Design review of the part built by this model. Coordinates are the model's own, in mm. A direction names the side the tool comes from. Coordinates: 2 decimals unless noted, no trailing zeros. Loops run counter-clockwise (first coordinate to the right, second up) from the corner with the lowest first, then second, coordinate; pieces in that order, holes last. Notation, with made-up numbers: M -24.5,31 L -1.5,31 A17 cw -1.5,60 Z; hole C 0,44.5 d4. An arc over 180 degrees is marked long. One line per item, written item: value.
```python
from build123d import *

# Parameters (mm, degrees)
BOSS_EXTRUDE1_DEPTH      = 14
BOSS_EXTRUDE1_DEPTH_BACK = 14
BOSS_EXTRUDE3_DEPTH      = 14.084146884
CUT_EXTRUDE1_START       = 11.1
CUT_EXTRUDE1_DEPTH       = 22.2
SKETCH7_R                = 8.05
CUT_EXTRUDE2_DEPTH       = 3
SKETCH8_R                = 3
CUT_EXTRUDE4_DEPTH       = 50.90760018
FILLET4_R                = 2
CHAMFER6_SIZE            = 1


with BuildPart() as part:
    # Sketch1 → Boss-Extrude1 (new, two sides: drawn at the far end of the back side and taken through both)
    with BuildSketch(Plane(origin=(0, 0, 0), x_dir=(0, 0, -1), z_dir=(1, 0, 0)).offset(-BOSS_EXTRUDE1_DEPTH_BACK)):
        Polygon((0, 0), (14.084146884, 0), (14.084146884, 26.488427786), align=None)
    extrude(amount=BOSS_EXTRUDE1_DEPTH + BOSS_EXTRUDE1_DEPTH_BACK)

    # Sketch5 → Boss-Extrude3 (add)
    with BuildSketch(Plane.XY):
        Polygon((14, -10), (14, 0), (11.1, 0), (11.1, -14), (31, -14), (31, -10), align=None)
        Polygon((-14, 0), (-14, -10), (-31, -10), (-31, -14), (-11.1, -14), (-11.1, 0), align=None)
    extrude(amount=-BOSS_EXTRUDE3_DEPTH)

    # Sketch6 → Cut-Extrude1 (cut)
    with BuildSketch(Plane(origin=(0, 0, 0), x_dir=(0, 0, -1), z_dir=(1, 0, 0)).offset(CUT_EXTRUDE1_START)):
        Polygon((14.084146884, 0), (2.126837727, 0), (14.084146884, 22.488427786), align=None)
    extrude(amount=-CUT_EXTRUDE1_DEPTH, mode=Mode.SUBTRACT)

    # Sketch7 → Cut-Extrude2 (cut)
    with BuildSketch(Plane(origin=(0, 0, 0), x_dir=(1, 0, 0), z_dir=(0, 0.4694715627858856, 0.8829475928589298))):
        with Locations(Location((0, 15, 0), (0, 0, 270))):
            Circle(SKETCH7_R)
    extrude(amount=-CUT_EXTRUDE2_DEPTH, mode=Mode.SUBTRACT)

    # Sketch8 → Cut-Extrude4 (cut, through all)
    with BuildSketch(Plane(origin=(0, -10, 0), x_dir=(1, 0, 0), z_dir=(0, 1, 0))):
        with Locations(Location((22, 7.042073442, 0), (0, 0, 270))):
            Circle(SKETCH8_R)
        with Locations(Location((-22, 7.042073442, 0), (0, 0, 90))):
            Circle(SKETCH8_R)
    extrude(amount=-CUT_EXTRUDE4_DEPTH, mode=Mode.SUBTRACT)

    # Fillet4
    fillet4_edges = [part.edges().sort_by_distance(p)[0] for p in [
        (14, -10, -7.042073442),
        (-14, -10, -7.042073442),
        (-11.1, 0, -1.063418863),
        (11.1, 0, -1.063418863),
        (11.1, 11.244213893, -8.105492305),
        (-11.1, 11.244213893, -8.105492305),
    ]]
    fillet(fillet4_edges, radius=FILLET4_R)

    # Chamfer6
    chamfer6_edges = [part.edges().sort_by_distance(p)[0] for p in [
        (14, 13.244213893, -7.042073442),
        (14.585786438, -9.414213562, 0),
        (14.585786438, -9.414213562, -14.084146884),
        (-14.585786438, -9.414213562, 0),
        (-14.585786438, -9.414213562, -14.084146884),
        (31, -10, -7.042073442),
        (14, -4, 0),
        (-31, -10, -7.042073442),
        (-14, -4, 0),
        (-14, 13.244213893, -7.042073442),
        (0, 20.351942015, -10.821319522),
        (23.5, -10, -14.084146884),
        (23.5, -10, 0),
        (14, 13.244213893, -14.084146884),
        (-14, 13.244213893, -14.084146884),
        (-23.5, -10, -14.084146884),
        (-23.5, -10, 0),
    ]]
    chamfer(chamfer6_edges, length=CHAMFER6_SIZE)


solid = part.part
```
(1) To check wall thickness, follow line 1 along X through (y, z) = (-1, -9); line 2 along Z through (x, y) = (-22, -11); line 3 along Y through (x, z) = (-25, -3). State the ranges of each line that lie inside material, in increasing order. Write a range as [from, to].
Reply:
line 1: x = [-14, -11.1], [11.1, 14]
line 2: z = [-14.08, -10.04], [-4.04, 0]
line 3: y = [-14, -10]
(2) We need section B-B on y = -7. State the section outline as (x, z) points.
Reply:
outline: M -14,-13.08 L -13,-14.08 L -11.1,-14.08 L -11.1,0 L -13,0 L -14,-1 Z; M 11.1,-14.08 L 13,-14.08 L 14,-13.08 L 14,-1 L 13,0 L 11.1,0 Z
(3) We need section C-C on x = 27. State the section outline as (y, z) points.
Reply:
outline: M -14,-14.08 L -11,-14.08 L -10,-13.08 L -10,-1 L -11,0 L -14,0 Z
(4) Tool access review of faces 1 (the flat face through (-26, -10, -7)), 2 (the cylindrical face through (-10.53, -0.6, -1.32)), 3 (the cylindrical face through (-10.53, 10.596, -8.442)): name each direction out of +Z, -Z, +X, -X, +Y, -Y from which nothing blocks a thin tool from reaching the whole face with its end or side.
Reply:
face 1: +Z, -Z, -X, +Y
face 2: +Z, -Z, -Y
face 3: -Z, -Y
(5) We need section A-A on x = -22. State the section outline as (y, z) points.
Reply:
outline: M -14,-14.08 L -11,-14.08 L -10,-13.08 L -10,-10.04 L -14,-10.04 Z; M -14,-4.04 L -10,-4.04 L -10,-1 L -11,0 L -14,0 Z
(6) Insertion check: pin 1 (7 mm diameter, centred on x = 22, z = -7.04, fed in from +Y); pin 2 (4 mm diameter, centred on y = -3, z = -8.5, fed in from +X); pin 3 (1 mm diameter, centred on x = 1, z = -4.5, fed in from -Y). Each pin has a flat end and moves straight along its axis. Give the tip position at first contact, or say it passes through.
Reply:
pin 1: stops at y = -10
pin 2: stops at x = 14
pin 3: stops at y = 3.52
(7) Mouldability with a two-part tool opening along X and no side actions: class faces 4 (the flat face through (25, -10, -6)), 5 (the flat face through (-11.1, -1, -9)), 6 (the cylindrical face through (10.499, 10.611, -8.415)), 7 (the flat face through (-14, 4, -8)) as released by +X, released by -X, zero draft, split by the parting line, or undercut.
Reply:
face 4: zero draft
face 5: undercut
face 6: undercut
face 7: released by -X
(8) We need section D-D on z = -7.5. State how many separate pieces and enclosed holes the cut face has, then the cut area to 3 significant figures.
Reply:
separate pieces: 4
enclosed holes: 0
area: 277 mm2
